```python
from build123d import *

# Parameters (mm, degrees)
SKETCH_1_W      = 20
SKETCH_1_H      = 20
EXTRUDE_1_DEPTH = 3
SKETCH_2_W      = 5
SKETCH_2_H      = 20
EXTRUDE_2_DEPTH = 3
SKETCH_3_W      = 5
SKETCH_3_H      = 3
EXTRUDE_3_DEPTH = 50
SKETCH_4_W      = 5
SKETCH_4_H      = 25
EXTRUDE_4_DEPTH = 30


with BuildPart() as part:
    # 草图1 → 凸台-拉伸1 (new body)
    with BuildSketch(Plane.XY):
        Rectangle(SKETCH_1_W, SKETCH_1_H)
    extrude(amount=EXTRUDE_1_DEPTH)

    # 草图2 → 凸台-拉伸2 (add)
    with BuildSketch(Plane.XY.offset(3)):
        Rectangle(SKETCH_2_W, SKETCH_2_H)
    extrude(amount=EXTRUDE_2_DEPTH)

    # 草图3 → 凸台-拉伸3 (add)
    with BuildSketch(Plane.XZ.offset(10)):
        with Locations((0, 4.5)):
            Rectangle(SKETCH_3_W, SKETCH_3_H)
    extrude(amount=EXTRUDE_3_DEPTH)

    # 草图4 → 凸台-拉伸4 (add)
    with BuildSketch(Plane.XY.offset(6)):
        with Locations((0, -47.5)):
            Rectangle(SKETCH_4_W, SKETCH_4_H)
    extrude(amount=EXTRUDE_4_DEPTH)


solid = part.part
```
The model under review builds one solid part; all positions refer to its coordinate system, in mm. A direction names the side the tool comes from. Round coordinates to 2 decimals unless told otherwise and drop trailing zeros. Order: outer loops, then holes, each group sorted by start corner. A loop starts at its lowest first (then second) coordinate and runs counter-clockwise, first axis right, second up. Notation, with made-up numbers: (-0.75, 50) -> (20.25, 50) arc R12 ccw to (20.25, 69) -> close; hole circle Ø5 at (53, -28.5). An arc over 180 degrees is marked (long way). Use a Markdown table: item, result.
Q1. Tool access review of faces 1 (the flat face through (6, 0, 3)), 2 (the flat face through (0, -10, 1)), 3 (the flat face through (-6, 0, 3)): name each direction out of +Z, -Z, +X, -X, +Y, -Y from which nothing blocks a thin tool from reaching the whole face with its end or side.
Values:
| item | result |
|---|---|
| face 1 | +Z, +X, +Y, -Y |
| face 2 | -Z, +X, -X, -Y |
| face 3 | +Z, -X, +Y, -Y |
Q2. We need section B-B on y = -22. Write out the cut boundary in (x, z).
Values:
| item | result |
|---|---|
| outline | (-2.5, 3) -> (2.5, 3) -> (2.5, 6) -> (-2.5, 6) -> close |
Q3. We need section A-A on x = 1. Write out the cut boundary in (y, z), then the cut area to 3 significant figures.
Values:
| item | result |
|---|---|
| outline | (-60, 3) -> (-10, 3) -> (-10, 0) -> (10, 0) -> (10, 6) -> (-35, 6) -> (-35, 36) -> (-60, 36) -> close |
| area | 1,020 mm^2 |
Q4. Clearance check with flat-ended pins moving along their axes: P1, Ø6, axis at x = 7, z = 23, coming from the +Y side; P2, Ø1.5, axis at x = 0, z = 27, coming from the +Y side; P3, Ø12, axis at y = -46.5, z = 15.5, coming from the +X side; P4, Ø0.9, axis at x = -2.5, z = 1, coming from the -Y side. State where each tip first meets the part, or that it passes through.
Values:
| item | result |
|---|---|
| P1 | passes through |
| P2 | stops at y = -35 |
| P3 | stops at x = 2.5 |
| P4 | stops at y = -10 |
Q5. For line 1 (X direction, y = -56, z = 6.5); line 2 (Y direction, x = -1.75, z = 33.5); line 3 (Y direction, x = -4.5, z = 1.5), list the stretches that pass through material, from the lowest coordinate up.
Values:
| item | result |
|---|---|
| line 1 | x = -2.5 to 2.5 |
| line 2 | y = -60 to -35 |
| line 3 | y = -10 to 10 |
Q6. We need section C-C on z = 15.5. Write out the cut boundary in (x, y), then the cut area to 3 significant figures.
Values:
| item | result |
|---|---|
| outline | (-2.5, -60) -> (2.5, -60) -> (2.5, -35) -> (-2.5, -35) -> close |
| area | 125 mm^2 |
